For this review, take the finished solid that the model builds, in its own axes (mm). Coordinates: 2 decimals unless noted, no trailing zeros. Write each loop counter-clockwise with the first axis right and the second up, starting at its lowest first coordinate (ties: lowest second). Pieces come first, ordered by that corner, then holes. Notation, with made-up numbers: (40, -0.75) - (80, -0.75) arc R11 ccw to (80, 20.25) - close; hole circle Ø8 at (28, 64.5). An arc over 180 degrees is marked (long way). Use one line per item in the form item = value. Start each with the question number.
1) For L1, parallel to X at y = 1.7, z = -17.5; L2, parallel to X at y = 0.75, z = -3.5; L3, parallel to Z at x = 65, y = 1.15, list the stretches that pass through material, from the lowest coordinate up. Write a range as from..to.
2) We need section C-C (y = 1.25). Count the separate pieces of the cut face and the enclosed holes in it, plus the area to 3 significant figures.
3) We need section B-B (x = 65). Give the boundary of the cut face in (y, z), plus the area to 3 significant figures.
4) We need section A-A (z = 17.5). Give the boundary of the cut face in (x, y), plus the area to 3 significant figures.
5) We need section D-D (z = 0). Give the boundary of the cut face in (x, y), plus the area to 4 significant figures.
6) Insertion check: P1, Ø2, axis at x = 20, z = -17.5, coming from the +Y side; P2, Ø0.8, axis at y = 1, z = -16, coming from the +X side. Each pin has a flat end and moves straight along its axis. Give the tip position at first contact, or say it passes through.
```python
from build123d import *

# Parameters (mm, degrees)
EXTRUDE_1_DEPTH     = 2.5
SKETCH_2_R          = 1.25
CUT_EXTRUDE_1_DEPTH = 78.661122835
SKETCH_3_R          = 2
CUT_EXTRUDE_2_DEPTH = 10


with BuildPart() as part:
    # 草图1 → 凸台-拉伸1 (new body)
    with BuildSketch(Plane(origin=(0, 0, 0), x_dir=(1, 0, 0), z_dir=(0, 1, 0))):
        Polygon((0, -20), (0, 20), (25, 20), (25, 5), (75, 5), (75, -5), (25, -5), (25, -20), align=None)
    extrude(amount=EXTRUDE_1_DEPTH)

    # 草图2 → 切除-拉伸1 (cut, through all)
    with BuildSketch(Plane(origin=(0, 0, 0), x_dir=(1, 0, 0), z_dir=(0, 1, 0))):
        with Locations(Location((10, 17.5, 0), (0, 0, 270))):
            Circle(SKETCH_2_R)
        with Locations(Location((20, 17.5, 0), (0, 0, 270))):
            Circle(SKETCH_2_R)
        with Locations(Location((20, 10.5, 0), (0, 0, 270))):
            Circle(SKETCH_2_R)
        with Locations(Location((20, 3.5, 0), (0, 0, 270))):
            Circle(SKETCH_2_R)
        with Locations(Location((20, -3.5, 0), (0, 0, 270))):
            Circle(SKETCH_2_R)
        with Locations(Location((20, -10.5, 0), (0, 0, 270))):
            Circle(SKETCH_2_R)
        with Locations(Location((20, -17.5, 0), (0, 0, 270))):
            Circle(SKETCH_2_R)
        with Locations(Location((10, 10.5, 0), (0, 0, 270))):
            Circle(SKETCH_2_R)
        with Locations(Location((10, 3.5, 0), (0, 0, 270))):
            Circle(SKETCH_2_R)
        with Locations(Location((10, -3.5, 0), (0, 0, 270))):
            Circle(SKETCH_2_R)
        with Locations(Location((10, -10.5, 0), (0, 0, 270))):
            Circle(SKETCH_2_R)
        with Locations(Location((10, -17.5, 0), (0, 0, 270))):
            Circle(SKETCH_2_R)
    extrude(amount=CUT_EXTRUDE_1_DEPTH, mode=Mode.SUBTRACT)

    # 草图3 → 切除-拉伸2 (cut)
    with BuildSketch(Plane(origin=(0, 0, 0), x_dir=(1, 0, 0), z_dir=(0, 1, 0))):
        with Locations(Location((65, 0, 0), (0, 0, 270))):
            Circle(SKETCH_3_R)
    extrude(amount=CUT_EXTRUDE_2_DEPTH, mode=Mode.SUBTRACT)


solid = part.part
```
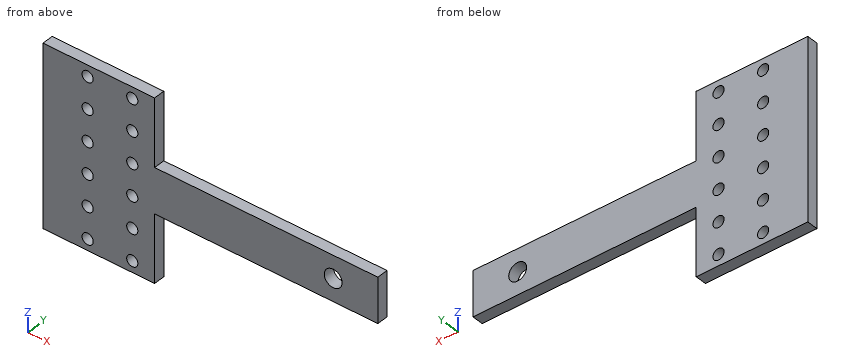
Determined:
q1.L1 = 0..8.75, 11.25..18.75, 21.25..25
q1.L2 = 0..8.75, 11.25..18.75, 21.25..75
q1.L3 = -5..-2, 2..5
q2.separate_pieces = 1
q2.enclosed_holes = 13
q2.area = 1,430 mm²
q3.outline = (0, -5) - (2.5, -5) - (2.5, -2) - (0, -2) - close; (0, 2) - (2.5, 2) - (2.5, 5) - (0, 5) - close
q3.area = 15.0 mm²
q4.outline = (0, 0) - (8.75, 0) - (8.75, 2.5) - (0, 2.5) - close; (11.25, 0) - (18.75, 0) - (18.75, 2.5) - (11.25, 2.5) - close; (21.25, 0) - (25, 0) - (25, 2.5) - (21.25, 2.5) - close
q4.area = 50.0 mm²
q5.outline = (0, 0) - (63, 0) - (63, 2.5) - (0, 2.5) - close; (67, 0) - (75, 0) - (75, 2.5) - (67, 2.5) - close
q5.area = 177.5 mm²
q6.P1 = through
q6.P2 = 25
